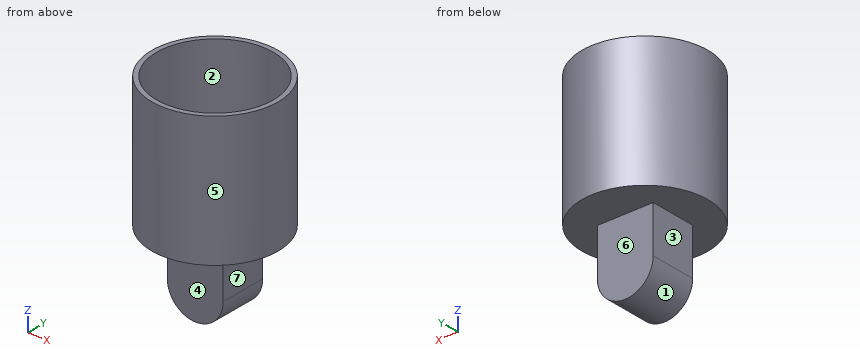
from build123d import *

# Parameters (mm, degrees)
SKETCH_1_R           = 13.5
SKETCH_1_R_2         = 12.5
EXTRUDE_1_DEPTH      = 25
SKETCH_2_R           = 13.5
EXTRUDE_2_DEPTH      = 3
EXTRUDE_3_DEPTH      = 5
EXTRUDE_3_DEPTH_BACK = 5


with BuildPart() as part:
    # Sketch 1 → Extrude 1 (new body)
    with BuildSketch(Plane.XY):
        Circle(SKETCH_1_R)
        Circle(SKETCH_1_R_2, mode=Mode.SUBTRACT)
    extrude(amount=-EXTRUDE_1_DEPTH)

    # Sketch 2 → Extrude 2 (add)
    with BuildSketch(Plane(origin=(0, 0, -25), x_dir=(-1, 0, 0), z_dir=(0, 0, -1))):
        with Locations(Location((0, 0, 0), (0, 0, 180))):
            Circle(SKETCH_2_R)
    extrude(amount=EXTRUDE_2_DEPTH)

    # Sketch 3 → Extrude 3 (add, two sides: drawn at the far end of the back side and taken through both)
    with BuildSketch(Plane(origin=(0, 0, 0), x_dir=(1, 0, 0), z_dir=(0, 1, 0)).offset(-EXTRUDE_3_DEPTH_BACK)):
        with BuildLine():
            Line((-6, 28), (6, 28))
            Line((6, 28), (6, 38))
            ThreePointArc((6, 38), (0, 44), (-6, 38))
            Line((-6, 38), (-6, 28))
        make_face()
    extrude(amount=EXTRUDE_3_DEPTH + EXTRUDE_3_DEPTH_BACK)


solid = part.part
Read the model definition and answer for the solid it produces. Units are mm, in the model's axes. Face numbers are marked on the shaded views. A direction names the side the tool comes from. Coordinates: 2 decimals unless noted, no trailing zeros. Order: outer loops, then holes, each group sorted by start corner. A loop starts at its lowest first (then second) coordinate and runs counter-clockwise, first axis right, second up. Notation, with made-up numbers: (79.25, 18) - (105.25, 18) arc R23 cw to (105.25, 50) - close; hole circle Ø1 at (77, 54.5). An arc over 180 degrees is marked (long way). Use one line per item in the form item = value.
(1) For a pull along X with two mould halves and no side action, classify the marked faces 1, 2 and 3 as pulls with the +X half, pulls with the -X half, needs draft (parallel to the pull), parting line crosses it, or undercut.
Computed values:
face_1 = parting line crosses it
face_2 = undercut
face_3 = pulls with the -X half
(2) Section C-C, the plane z = -7.5 is taken. Give the vertices of the cut face in (x, y).
Computed values:
outline = circle Ø27 at (0, 0); hole circle Ø25 at (0, 0)
(3) Section B-B, the plane x = 0 is taken. Give the vertices of the cut face in (y, z).
Computed values:
outline = (-13.5, -28) - (-5, -28) - (-5, -44) - (5, -44) - (5, -28) - (13.5, -28) - (13.5, 0) - (12.5, 0) - (12.5, -25) - (-12.5, -25) - (-12.5, 0) - (-13.5, 0) - close
(4) Section D-D, the plane y = -9.75 is taken. Give the vertices of the cut face in (x, z).
Computed values:
outline = (-9.34, -28) - (9.34, -28) - (9.34, 0) - (7.82, 0) - (7.82, -25) - (-7.82, -25) - (-7.82, 0) - (-9.34, 0) - close
(5) Section A-A, the plane y = 0 is taken. Give the vertices of the cut face in (x, z).
Computed values:
outline = (-13.5, -28) - (-6, -28) - (-6, -38) arc R6 ccw to (6, -38) - (6, -28) - (13.5, -28) - (13.5, 0) - (12.5, 0) - (12.5, -25) - (-12.5, -25) - (-12.5, 0) - (-13.5, 0) - close
(6) Given pin 1 Ø10 at (y, z) = (7.5, -14) entering from +X; pin 2 Ø1.5 at (x, y) = (10, -2.5) entering from -Z; pin 3 Ø9.5 at (x, z) = (3, -34) entering from +Y, each flat-ended and moving along its own axis, determine where each tip first touches the part or whether it passes through.
Computed values:
pin_1 = 13.27
pin_2 = -28
pin_3 = 5
(7) Which of the six approach directions +Z, -Z, +X, -X, +Y, -Y give full straight-line access (tool end or side, diameter ignored) to the marked faces 4, 5, 6 and 7?
Computed values:
face_4 = -Z, +X, -X, -Y
face_5 = +Z, -Z
face_6 = -Z, +X, -X, +Y
face_7 = -Z, +X, +Y, -Y
(8) Straight lines are drawn through the part: L1, parallel to Y at x = 0, z = -11.5; L2, parallel to X at y = 0.5, z = -2.5; L3, parallel to Z at x = -8, y = 3.25. For each, find the intervals that lie inside material, in ascending order.
Computed values:
L1 = -13.5 to -12.5, 12.5 to 13.5
L2 = -13.49 to -12.49, 12.49 to 13.49
L3 = -28 to -25
